```python
from build123d import *

# Parameters (mm, degrees)
BOSS_EXTRU_1_DEPTH      = 2
ENL_V_MAT_EXTRU_1_DEPTH = 10
ESQUISSE3_R             = 1.52
ENL_V_MAT_EXTRU_2_DEPTH = 10


with BuildPart() as part:
    # Esquisse1 → Boss.-Extru.1 (new body)
    with BuildSketch(Plane.XY):
        with BuildLine():
            Line((-69.5, -97.5), (69.5, -97.5))
            ThreePointArc((69.5, -97.5), (71.621320344, -96.621320344), (72.5, -94.5))
            Line((72.5, -94.5), (72.5, 99.5))
            ThreePointArc((72.5, 99.5), (71.621320344, 101.621320344), (69.5, 102.5))
            Line((69.5, 102.5), (-69.5, 102.5))
            ThreePointArc((-69.5, 102.5), (-71.621320344, 101.621320344), (-72.5, 99.5))
            Line((-72.5, 99.5), (-72.5, -94.5))
            ThreePointArc((-72.5, -94.5), (-71.621320344, -96.621320344), (-69.5, -97.5))
        make_face()
    extrude(amount=BOSS_EXTRU_1_DEPTH)

    # Esquisse2 → Enlèv. mat.-Extru.1 (cut)
    with BuildSketch(Plane(origin=(0, 0, 0), x_dir=(-1, 0, 0), z_dir=(0, 0, -1))):
        with BuildLine():
            Line((-27.945607011, -41.449532586), (28.054392989, -41.449532586))
            ThreePointArc((28.054392989, -41.449532586), (29.468606552, -40.863746148), (30.054392989, -39.449532586))
            Line((30.054392989, -39.449532586), (30.054392989, 16.550467414))
            ThreePointArc((30.054392989, 16.550467414), (29.468606552, 17.964680976), (28.054392989, 18.550467414))
            Line((28.054392989, 18.550467414), (-27.945607011, 18.550467414))
            ThreePointArc((-27.945607011, 18.550467414), (-29.359820573, 17.964680976), (-29.945607011, 16.550467414))
            Line((-29.945607011, 16.550467414), (-29.945607011, -39.449532586))
            ThreePointArc((-29.945607011, -39.449532586), (-29.359820573, -40.863746148), (-27.945607011, -41.449532586))
        make_face()
    extrude(amount=-ENL_V_MAT_EXTRU_1_DEPTH, mode=Mode.SUBTRACT)

    # Esquisse3 → Enlèv. mat.-Extru.2 (cut)
    with BuildSketch(Plane.XY.offset(2)):
        with Locations((69.5, 99.5)):
            Circle(ESQUISSE3_R)
        with Locations((-69.5, 99.5)):
            Circle(ESQUISSE3_R)
        with Locations((-69.5, -94.5)):
            Circle(ESQUISSE3_R)
        with Locations((69.5, -94.5)):
            Circle(ESQUISSE3_R)
    extrude(amount=-ENL_V_MAT_EXTRU_2_DEPTH, mode=Mode.SUBTRACT)


solid = part.part
```
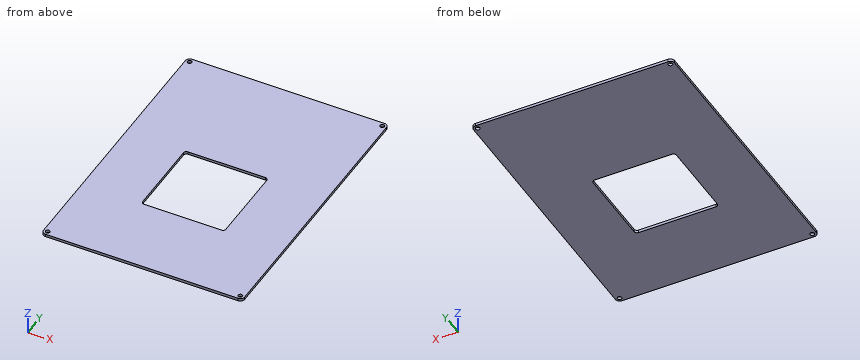
Design review of the part built by this model. Coordinates are the model's own, in mm. Coordinates: 2 decimals unless noted, no trailing zeros. Order: outer loops, then holes, each group sorted by start corner. A loop starts at its lowest first (then second) coordinate and runs counter-clockwise, first axis right, second up.
1) Clearance check with flat-ended pins moving along their axes: pin 1 (8 mm diameter, centred on x = 54.5, y = 49, fed in from -Z); pin 2 (1.8 mm diameter, centred on x = 69.5, y = 99.5, fed in from -Z). State where each tip first meets the part, or that it passes through.
2) Take a section at A-A, the plane x = -1.5. Give the boundary of the cut face in (y, z), and give its area (3 significant figures).
3) Wall thickness on line 1 along X through (y, z) = (-94.5, 1.15); line 2 along Y through (x, z) = (69.5, 0.8); line 3 along Y through (x, z) = (-6.5, 1.8): over which ranges is each line inside the solid? List them lowest first.
4) Take a section at B-B, the plane z = 1.1. Give the boundary of the cut face in (x, y), and give its area (3 significant figures).
Returned:
1. pin 1: stops at z = 0
1. pin 2: passes through
2. outline: (-97.5, 0) - (-41.45, 0) - (-41.45, 2) - (-97.5, 2) - close; (18.55, 0) - (102.5, 0) - (102.5, 2) - (18.55, 2) - close
2. area: 280 mm2
3. line 1: x = -72.5 to -71.02, -67.98 to 67.98, 71.02 to 72.5
3. line 2: y = -97.5 to -96.02, -92.98 to 97.98, 101.02 to 102.5
3. line 3: y = -97.5 to -41.45, 18.55 to 102.5
4. outline: (-72.5, -94.5) arc R3 ccw to (-69.5, -97.5) - (69.5, -97.5) arc R3 ccw to (72.5, -94.5) - (72.5, 99.5) arc R3 ccw to (69.5, 102.5) - (-69.5, 102.5) arc R3 ccw to (-72.5, 99.5) - close; hole circle Ø3.04 at (-69.5, -94.5); hole circle Ø3.04 at (-69.5, 99.5); hole (-30.05, -39.45) arc R2 ccw to (-28.05, -41.45) - (27.95, -41.45) arc R2 ccw to (29.95, -39.45) - (29.95, 16.55) arc R2 ccw to (27.95, 18.55) - (-28.05, 18.55) arc R2 ccw to (-30.05, 16.55) - close; hole circle Ø3.04 at (69.5, -94.5); hole circle Ø3.04 at (69.5, 99.5)
4. area: 25,400 mm2
